Read the model definition and answer for the solid it produces. Units are mm, in the model's axes. Face numbers are marked on the shaded views. A direction names the side the tool comes from. Give positions to 0.01 mm unless a question says otherwise; leave off trailing zeros. Order: outer loops, then holes, each group sorted by start corner. A loop starts at its lowest first (then second) coordinate and runs counter-clockwise, first axis right, second up. Notation, with made-up numbers: M 80,69.5 L 121,69.5 A21 ccw 121,88.5 Z; hole C -38.5,63.5 d8. An arc over 180 degrees is marked long. One line per item, written item: value. Start each with the question number.
from build123d import *
from build123d.topology import SkipClean

# Parameters (mm, degrees)
SKETCH1_R           = 2.75
BOSS_EXTRUDE1_DEPTH = 22.5
BOSS_EXTRUDE2_START = 1.5
BOSS_EXTRUDE2_DEPTH = 1.5
BOSS_EXTRUDE3_DEPTH = 1.5
SKETCH5_W           = 25.5
SKETCH5_H           = 5.5
BOSS_EXTRUDE4_DEPTH = 1.5
CUT_EXTRUDE1_DEPTH  = 0.5


with BuildPart() as part:
    # Sketch1 → Boss-Extrude1 (new body)
    with BuildSketch(Plane(origin=(0, 0, 0), x_dir=(0, 0, -1), z_dir=(1, 0, 0))):
        with Locations(Location((0, 0, 0), (0, 0, 180))):
            Circle(SKETCH1_R)
    extrude(amount=BOSS_EXTRUDE1_DEPTH)

    # Sketch2 → Boss-Extrude2 (add)
    with SkipClean():  # the faces are left unmerged after this step: merging them gives an invalid solid
        with BuildSketch(Plane.ZY.offset(BOSS_EXTRUDE2_START)):
            with BuildLine():
                Line((0, 2.75), (-17.25, 2.75))
                Line((-17.25, 2.75), (-17.25, -2.75))
                Line((-17.25, -2.75), (0, -2.75))
                ThreePointArc((0, -2.75), (2.75, 0), (0, 2.75))
            make_face()
        extrude(amount=-BOSS_EXTRUDE2_DEPTH)

    # Sketch3 → Boss-Extrude3 (add)
    with BuildSketch(Plane(origin=(22.5, 0, 0), x_dir=(0, 0, -1), z_dir=(1, 0, 0))):
        with BuildLine():
            Line((0, -2.75), (17.25, -2.75))
            Line((17.25, -2.75), (17.25, 2.75))
            Line((17.25, 2.75), (0, 2.75))
            ThreePointArc((0, 2.75), (-2.75, 0), (0, -2.75))
        make_face()
    extrude(amount=BOSS_EXTRUDE3_DEPTH)

    # Sketch5 → Boss-Extrude4 (add)
    with BuildSketch(Plane(origin=(0, 0, -17.25), x_dir=(-1, 0, 0), z_dir=(0, 0, -1))):
        with Locations((-11.25, 0)):
            Rectangle(SKETCH5_W, SKETCH5_H)
    extrude(amount=BOSS_EXTRUDE4_DEPTH)

    # Sketch6 → Cut-Extrude1 (cut)
    with BuildSketch(Plane(origin=(0, 2.75, 0), x_dir=(1, 0, 0), z_dir=(0, 1, 0))):
        with BuildLine():
            Line((10.25, 17.25), (10.25, 0))
            Line((10.25, 0), (12.25, 0))
            Line((12.25, 0), (12.25, 17.25))
            ThreePointArc((12.25, 17.25), (11.25, 18.25), (10.25, 17.25))
        make_face()
    extrude(amount=-CUT_EXTRUDE1_DEPTH, mode=Mode.SUBTRACT)


solid = part.part
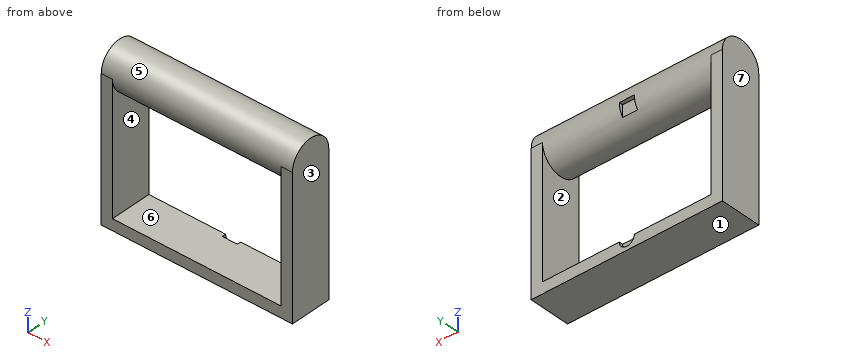
Q1. A tool of negligible diameter and unlimited length cuts with its end or side. For the marked faces 5, 6 and 7, from which of +Z, -Z, +X, -X, +Y, -Y can it reach the whole face along a straight path? Write none if from no direction.
Q2. Each of these flat-tipped pins is pushed along its axis until it touches: pin 1 (12 mm diameter, centred on x = 18, z = -9, fed in from +Y); pin 2 (1.6 mm diameter, centred on x = 7.5, y = 1.5, fed in from +Z); pin 3 (0.5 mm diameter, centred on x = 11, z = -0.5, fed in from +Y). Where does it stop, or does it pass through?
Q3. Find section D-D, the plane x = 19. Give the vertices of the cut face in (y, z).
Q4. Find section A-A, the plane z = -10. Give the vertices of the cut face in (x, y).
Q5. Find section C-C, the plane y = 0. Give the vertices of the cut face in (x, z), then the cut area to 3 significant figures.
Q6. Determine the mould class of the marked faces 1, 2, 3 and 4 for opening direction Z: released by +Z, released by -Z, zero draft, split by the parting line, or undercut.
Q7. Consider probe 1 along X at (y, z) = (2.2, -16.75); probe 2 along Z at (x, y) = (11.5, 0.15); probe 3 along Z at (x, y) = (6, 1.75). Determine where each line is inside the solid, lowest interval first.
Q8. Find section B-B, the plane x = 11.25. Give the vertices of the cut face in (y, z).
Evaluation:
1. face 5: none
1. face 6: +Y, -Y
1. face 7: +Z, -Z, -X, +Y, -Y
2. pin 1: y = 2.75
2. pin 2: z = 2.66
2. pin 3: y = 2.25
3. outline: M -2.75,-18.75 L 2.75,-18.75 L 2.75,-17.25 L -2.75,-17.25 Z; C 0,0 d5.5
4. outline: M -1.5,-2.75 L 0,-2.75 L 0,2.75 L -1.5,2.75 Z; M 22.5,-2.75 L 24,-2.75 L 24,2.75 L 22.5,2.75 Z
5. outline: M -1.5,-18.75 L 24,-18.75 L 24,2.75 L -1.5,2.75 Z; hole M 0,-17.25 L 22.5,-17.25 L 22.5,-2.75 L 0,-2.75 Z
5. area: 222 mm2
6. face 1: released by -Z
6. face 2: undercut
6. face 3: zero draft
6. face 4: undercut
7. probe 1: -1.5 to 0, 22.5 to 24
7. probe 2: -18.75 to -17.25, -2.75 to 2.75
7. probe 3: -18.75 to -17.25, -2.12 to 2.12
8. outline: M -2.75,-18.75 L 2.75,-18.75 L 2.75,-18.25 L 2.25,-18.25 L 2.25,-17.25 L -2.75,-17.25 Z; M 2.25,-1.58 L 2.25,0 L 2.75,0 A2.75 ccw long Z
